Geometry check sheet. Reference: the model listing, model coordinates, mm. Face numbers are marked on the shaded views. A direction names the side the tool comes from. Coordinates: 2 decimals unless noted, no trailing zeros. Write each loop counter-clockwise with the first axis right and the second up, starting at its lowest first coordinate (ties: lowest second). Pieces come first, ordered by that corner, then holes. Notation, with made-up numbers: M 13.25,20 L 32.25,20 A19 ccw 32.25,52 Z; hole C 71,-1.5 d9. An arc over 180 degrees is marked long. Put each result on its own line as item: value. Start each with the question number.
1) Cross-section at C-C on x = -878. Record the cut outline in (y, z), plus the area to 3 significant figures.
2) Cross-section at A-A on z = 211. Record the cut outline in (x, y).
3) Scan lines: line 1 along Y through (x, z) = (-1195, 355.5); line 2 along Z through (x, y) = (-914.4, 705); line 3 along X through (y, z) = (315, 401.5). Record each from-to range of solid material in increasing order.
4) Cross-section at D-D on y = 390.5. Record the cut outline in (x, z), plus the area to 3 significant figures.
5) Cross-section at B-B on y = -5.5. Record the cut outline in (x, z), plus the area to 3 significant figures.
6) Set-up check for the marked faces 5, 6 and 7: record each of +Z, -Z, +X, -X, +Y, -Y from which the full face is reachable in a straight line by a thin tool's end or side.
7) Mould release check, pull along Z, two halves, no side actions. Record for the marked faces 1, 2, 3 and 4: released by +Z, released by -Z, zero draft, split by the parting line, or undercut.
8) Gauge pin test, flat ends, axial feed: pin 1 (1.5 mm diameter, centred on y = 632, z = 595.5, fed in from -X); pin 2 (3 mm diameter, centred on y = 192, z = 596.5, fed in from -X); pin 3 (1.5 mm diameter, centred on y = 697.5, z = 614.5, fed in from -X). Record the tip position at first contact, or that the pin passes through.
from build123d import *
from build123d import SkipClean  # not in build123d's __all__

# Parameters (mm, degrees)
F0_R      = 228.6
F1_DEPTH  = 812.8
F0_W      = 1016
F0_H      = 812.8
F1_FACE_R = 228.6
F2_DEPTH  = 914.4
F4_DEPTH  = 279.4
F6_DEPTH  = 1016.001
F7_W      = 635
F7_H      = 457.2
F8_DEPTH  = 812.801
F10_DEPTH = 279.4


# Not quite as in the source:
# - after a boolean that leaves OpenCascade's solid faulty, fix() repairs it


with BuildPart() as f1:
    # F0 (on Right) → F1 (new body)
    with BuildSketch(Plane.YZ):
        with Locations((330.030798912, 303.7791848183)):
            Circle(F0_R)
    extrude(amount=F1_DEPTH)

    # F0 (on Right) + F1_face (on face) → F2 (join)
    with BuildSketch(Plane.YZ):
        with Locations((384.9944980741, 337.2235123754)):
            Rectangle(F0_W, F0_H)
        with Locations((330.030798912, 303.7791848183)):
            Circle(F0_R, mode=Mode.SUBTRACT)
    with BuildSketch(Plane(origin=(0, 330.030798912, 303.7791848183), x_dir=(0, 1, 0), z_dir=(-1, 0, 0))):
        Circle(F1_FACE_R)
    extrude(amount=-F2_DEPTH, dir=(1, 0, 0))

    # F3 (on face) → F4 (join)
    with BuildSketch(Plane.XZ.offset(123.0055019259)):
        with BuildLine():
            ThreePointArc((-914.4, 743.6235123754), (-1320.8, 337.2235123754), (-914.4, -69.1764876246))
            Line((-914.4, -69.1764876246), (-914.4, 134.0235123754))
            ThreePointArc((-914.4, 134.0235123754), (-1117.6, 337.2235123754), (-914.4, 540.4235123754))
            Line((-914.4, 540.4235123754), (-914.4, 743.6235123754))
        make_face()
    extrude(amount=-F4_DEPTH)

    # F5 (on face) → F6 (cut, through all)
    with BuildSketch(Plane.XZ.offset(123.0055019259)):
        with BuildLine():
            Line((-914.4, 540.4235123754), (-914.4, 134.0235123754))
            ThreePointArc((-914.4, 134.0235123754), (-770.7159020629, 193.5394144382), (-711.2, 337.2235123754))
            ThreePointArc((-711.2, 337.2235123754), (-770.7159020629, 480.9076103125), (-914.4, 540.4235123754))
        make_face()
    with SkipClean():  # cleaning this boolean's faces spoils the solid; the shape is the same uncleaned
        extrude(amount=-F6_DEPTH, mode=Mode.SUBTRACT)

    # F7 (on face) → F8 (cut, through all)
    with BuildSketch(Plane.XY.offset(743.6235123754)):
        with Locations((-596.9, 384.9944980741)):
            Rectangle(F7_W, F7_H)
    extrude(amount=-F8_DEPTH, mode=Mode.SUBTRACT)

    add(f1.part.fix(), mode=Mode.REPLACE)

    # F9 (on face) → F10 (join)
    with BuildSketch(Plane.XZ.offset(-613.5944980741)):
        with BuildLine():
            Line((-914.4, 540.4235123754), (-914.4, 743.6235123754))
            ThreePointArc((-914.4, 743.6235123754), (-1320.8, 337.2235123754), (-914.4, -69.1764876246))
            Line((-914.4, -69.1764876246), (-914.4, 134.0235123754))
            ThreePointArc((-914.4, 134.0235123754), (-1117.6, 337.2235123754), (-914.4, 540.4235123754))
        make_face()
    extrude(amount=-F10_DEPTH)


solid = f1.part
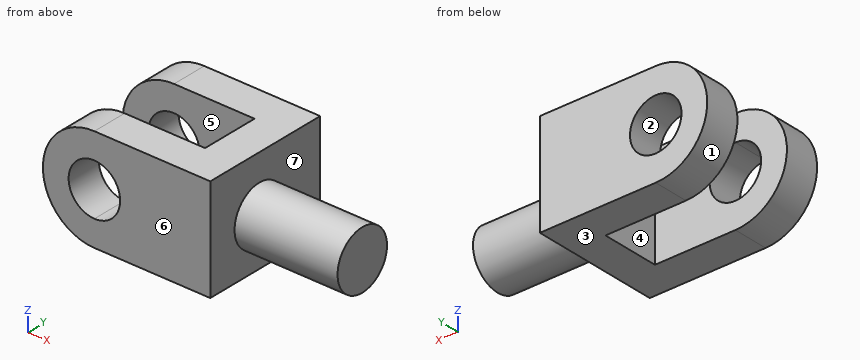
Answer key:
1. outline: M -123.01,-69.18 L 156.39,-69.18 L 156.39,137.31 L -123.01,137.31 Z; M -123.01,537.14 L 156.39,537.14 L 156.39,743.62 L -123.01,743.62 Z; M 613.59,-69.18 L 892.99,-69.18 L 892.99,137.31 L 613.59,137.31 Z; M 613.59,537.14 L 892.99,537.14 L 892.99,743.62 L 613.59,743.62 Z
1. area: 231,000 mm²
2. outline: M -1300.7,-123.01 L -1073.64,-123.01 L -1073.64,156.39 L -1300.7,156.39 Z; M -1300.7,613.59 L -1073.64,613.59 L -1073.64,892.99 L -1300.7,892.99 Z; M -755.16,-123.01 L 0,-123.01 L 0,121.11 L 812.8,121.11 L 812.8,538.96 L 0,538.96 L 0,892.99 L -755.16,892.99 L -755.16,613.59 L -279.4,613.59 L -279.4,156.39 L -755.16,156.39 Z
3. line 1: y = -123.01 to 156.39, 613.59 to 892.99
3. line 2: z = -69.18 to 134.02, 540.42 to 743.62
3. line 3: x = -279.4 to 812.8
4. outline: M -279.4,-69.18 L 0,-69.18 L 0,83.32 L 812.8,83.32 L 812.8,524.24 L 0,524.24 L 0,743.62 L -279.4,743.62 Z
4. area: 585,000 mm²
5. outline: M -914.4,-69.18 L 0,-69.18 L 0,743.62 L -914.4,743.62 A406.4 ccw Z; hole C -914.4,337.22 d406.4
5. area: 873,000 mm²
6. face 5: +Z, -Z, -X
6. face 6: +Z, -Z, +X, -X, -Y
6. face 7: +X
7. face 1: split by the parting line
7. face 2: undercut
7. face 3: released by -Z
7. face 4: zero draft
8. pin 1: stops at x = -1228.79
8. pin 2: stops at x = -279.4
8. pin 3: stops at x = -1212.22
